from build123d import *

# Parameters (mm, degrees)
F0_W     = 78.710422
F0_H     = 78.577757
F1_DEPTH = 25.4
F3_DEPTH = 25.4
F5_DEPTH = 78.711422
F7_DEPTH = 78.578757


with BuildPart() as f1:
    # F0 (on Top) → F1 (new body)
    with BuildSketch(Plane.XY):
        with Locations((1.636606, 2.354868)):
            Rectangle(F0_W, F0_H)
    extrude(amount=F1_DEPTH)

    # F2 (on face) → F3 (cut)
    with BuildSketch(Plane.XY.offset(25.4)):
        Polygon((9.63136, -16.870158), (19.425666, -0.094076), (9.794305, 16.776082), (-9.63136, 16.870158), (-19.425666, 0.094076), (-9.794305, -16.776082), align=None)
    extrude(amount=-F3_DEPTH, mode=Mode.SUBTRACT)

    # F4 (on face) → F5 (cut, through all)
    with BuildSketch(Plane(origin=(-37.718605, 0, 0), x_dir=(0, -1, 0), z_dir=(-1, 0, 0))):
        Polygon((6.126571, 16.465323), (-0.017433, 19.992435), (-6.144003, 16.435129), (-6.126571, 9.35071), (0.017433, 5.823597), (6.144003, 9.380904), align=None)
    extrude(amount=-F5_DEPTH, mode=Mode.SUBTRACT)

    # F6 (on face) → F7 (cut, through all)
    with BuildSketch(Plane.XZ.offset(36.934011)):
        Polygon((6.207672, 9.324016), (6.207672, 16.492018), (0, 20.076019), (-6.207672, 16.492018), (-6.207672, 9.324016), (0, 5.740015), align=None)
    extrude(amount=-F7_DEPTH, mode=Mode.SUBTRACT)


solid = f1.part
Geometry: final body of the model. Coordinates: model frame, mm. A direction names the side the tool comes from. Give positions to 0.01 mm unless a question says otherwise; leave off trailing zeros. Order: outer loops, then holes, each group sorted by start corner. A loop starts at its lowest first (then second) coordinate and runs counter-clockwise, first axis right, second up. Notation, with made-up numbers: (-30, 23) -> (15, 23) arc R16 ccw to (15, 27) -> close; hole circle Ø4 at (65.5, -27). An arc over 180 degrees is marked (long way). Put each result on its own line as item: value.
Q1. Material intervals for L1, parallel to Y at x = -8, z = 1; L2, parallel to X at y = 4.5, z = 6.75; L3, parallel to X at y = 25.5, z = 12, sorted ascending.
Here are the results:
L1: y = -36.93 to -16.78, 16.86 to 41.64
L2: x = -37.72 to -16.85, 16.8 to 40.99
L3: x = -37.72 to -6.21, 6.21 to 40.99
Q2. Reachability of faces 4 (the face through (13.372, -10.464, 12.878)), 5 (the face through (6.208, 29, 13)), 6 (the face through (-26.964, 3.098, 7.612)) from +Z, -Z, +X, -X, +Y, -Y: full face, straight path, thin tool, end or side. Return the list, or none.
Here are the results:
face 4: +Z, -Z
face 5: +Y, -Y
face 6: +X, -X
Q3. Draft query along X for faces 1 (the face through (40.992, 2, 21)), 2 (the face through (28.272, -3.098, 18.204)), 3 (the face through (3.147, 29.045, 18.259)). Return one class per face: released by +X, released by -X, zero draft, split by the parting line, or undercut.
Here are the results:
face 1: released by +X
face 2: zero draft
face 3: undercut
Q4. Section B-B, the plane z = 2. Return loops of the section in (x, y).
Here are the results:
outline: (-37.72, -36.93) -> (40.99, -36.93) -> (40.99, 41.64) -> (-37.72, 41.64) -> close; hole (-19.43, 0.09) -> (-9.79, -16.78) -> (9.63, -16.87) -> (19.43, -0.09) -> (9.79, 16.78) -> (-9.63, 16.87) -> close
Q5. Section C-C, the plane y = -7.5. Return loops of the section in (x, z), then the cut area to 3 significant figures.
Here are the results:
outline: (-37.72, 0) -> (-15.09, 0) -> (-15.09, 25.4) -> (-37.72, 25.4) -> close; (15.1, 0) -> (40.99, 0) -> (40.99, 25.4) -> (15.1, 25.4) -> close
area: 1,230 mm^2
Q6. Section A-A, the plane x = -22.5. Return loops of the section in (y, z), then the cut area to 3 significant figures.
Here are the results:
outline: (-36.93, 0) -> (41.64, 0) -> (41.64, 25.4) -> (-36.93, 25.4) -> close; hole (-6.14, 9.38) -> (-0.02, 5.82) -> (6.13, 9.35) -> (6.14, 16.44) -> (0.02, 19.99) -> (-6.13, 16.47) -> close
area: 1,870 mm^2
Q7. Section D-D, the plane z = 7.75. Return loops of the section in (x, y), then the cut area to 3 significant figures.
Here are the results:
outline: (-37.72, -36.93) -> (-3.48, -36.93) -> (-3.48, -16.81) -> (-9.79, -16.78) -> (-17.47, -3.34) -> (-37.72, -3.34) -> close; (-37.72, 3.34) -> (-17.53, 3.34) -> (-9.63, 16.87) -> (-3.48, 16.84) -> (-3.48, 41.64) -> (-37.72, 41.64) -> close; (3.48, -36.93) -> (40.99, -36.93) -> (40.99, -3.34) -> (17.53, -3.34) -> (9.63, -16.87) -> (3.48, -16.84) -> close; (3.48, 16.81) -> (9.79, 16.78) -> (17.47, 3.34) -> (40.99, 3.34) -> (40.99, 41.64) -> (3.48, 41.64) -> close
area: 4,610 mm^2
